Geometry: see drawing. Coordinates: mm, zero at the bounding-box minimum. Round coordinates to 2 decimals unless told otherwise and drop trailing zeros. Loops run counter-clockwise (first coordinate to the right, second up) from the corner with the lowest first, then second, coordinate; pieces in that order, holes last. Notation, with made-up numbers: (38, 5) - (60, 5) arc R30 ccw to (60, 35) - close; hole circle Ø5 at (-38.5, 81). An arc over 180 degrees is marked (long way). Return JSON: item names as keys, results as strings. Group by question number.
1. Section D-D on z = 7.75. Return loops of the section in (x, y).
2. Draft query along Y for the marked faces 1, 2 and 3. Return one class per face: +Y half, -Y half, draft (parallel to the pull), parting line (faces both ways), or undercut.
3. Section B-B on y = 32.5. Return loops of the section in (x, z).
4. Section C-C on x = 46.5. Return loops of the section in (y, z) (1 decimal).
5. Section A-A on z = 2. Return loops of the section in (x, y) (1 decimal), and give its area (3 significant figures).
6. Material intervals for probe 1 along X at (y, z) = (9, 6) (1 decimal); probe 2 along X at (y, z) = (33.5, 1); probe 3 along Y at (x, z) = (7, 2.25), sorted ascending.
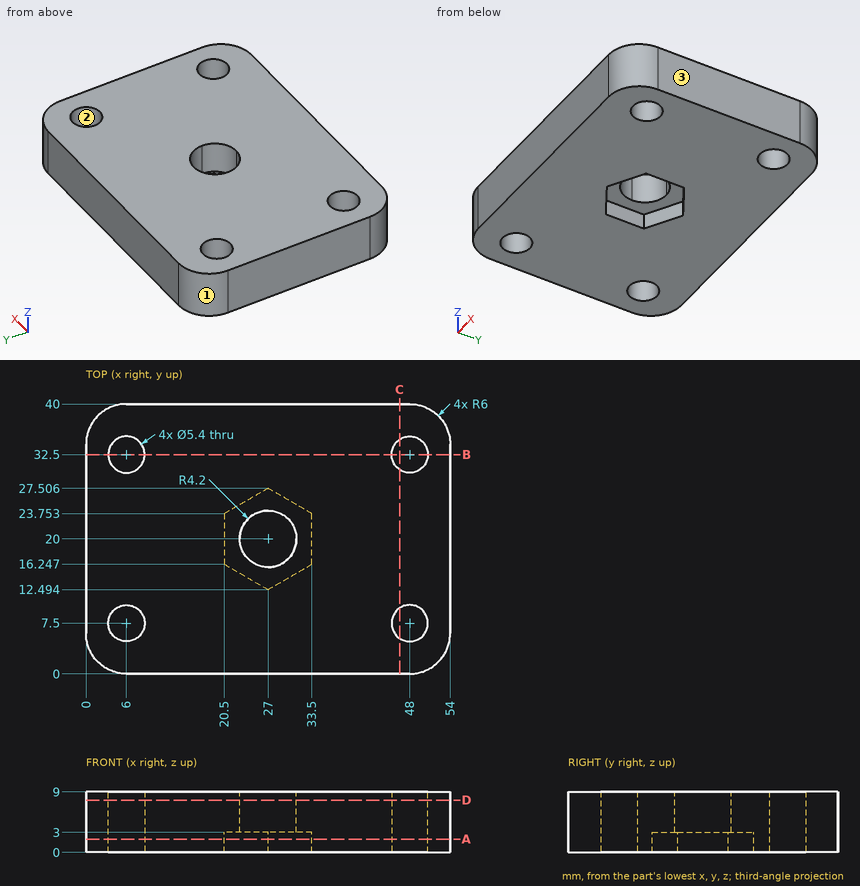
Taken from the geometry:
{
 "1": {"outline": "(0, 6) arc R6 ccw to (6, 0) - (48, 0) arc R6 ccw to (54, 6) - (54, 34) arc R6 ccw to (48, 40) - (6, 40) arc R6 ccw to (0, 34) - close; hole circle Ø5.4 at (6, 7.5); hole circle Ø5.4 at (6, 32.5); hole (22.8, 20) arc R4.2 ccw to (27, 15.8) arc R4.2 ccw to (31.2, 20) arc R4.2 ccw to (27, 24.2) arc R4.2 ccw to start; hole circle Ø5.4 at (48, 7.5); hole circle Ø5.4 at (48, 32.5)"},
 "2": {"face 1": "+Y half", "face 2": "undercut", "face 3": "draft"},
 "3": {"outline": "(0, 0) - (3.3, 0) - (3.3, 9) - (0, 9) - close; (8.7, 0) - (45.3, 0) - (45.3, 9) - (8.7, 9) - close; (50.7, 0) - (54, 0) - (54, 9) - (50.7, 9) - close"},
 "4": {"outline": "(0, 0) - (5.3, 0) - (5.3, 9) - (0, 9) - close; (9.7, 0) - (30.3, 0) - (30.3, 9) - (9.7, 9) - close; (34.7, 0) - (40, 0) - (40, 9) - (34.7, 9) - close"},
 "5": {"outline": "(0, 6) arc R6 ccw to (6, 0) - (48, 0) arc R6 ccw to (54, 6) - (54, 34) arc R6 ccw to (48, 40) - (6, 40) arc R6 ccw to (0, 34) - close; hole circle Ø5.4 at (6, 7.5); hole circle Ø5.4 at (6, 32.5); hole (20.5, 16.2) - (27, 12.5) - (33.5, 16.2) - (33.5, 23.8) - (27, 27.5) - (20.5, 23.8) - close; hole circle Ø5.4 at (48, 7.5); hole circle Ø5.4 at (48, 32.5)", "area": "1,890 mm2"},
 "6": {"probe 1": "0 to 3.8, 8.2 to 45.8, 50.2 to 54", "probe 2": "0 to 3.49, 8.51 to 45.49, 50.51 to 54", "probe 3": "0 to 4.99, 10.01 to 29.99, 35.01 to 40"}
}
